from build123d import *

# Parameters (mm, degrees)
BOSS_EXTRU_1_DEPTH      = 5
ESQUISSE2_W             = 5
ESQUISSE2_H             = 28
ESQUISSE2_W_2           = 47.6
ESQUISSE2_H_2           = 5
ESQUISSE2_H_3           = 33
ENL_V_MAT_EXTRU_1_DEPTH = 5


with BuildPart() as part:
    # Esquisse1 → Boss.-Extru.1 (new body)
    with BuildSketch(Plane.XY):
        Polygon((0, 0), (0, 145), (238, 170), (238, 5), (238, 0), align=None)
    extrude(amount=BOSS_EXTRU_1_DEPTH)

    # Esquisse2 → Enlèv. mat.-Extru.1 (cut)
    with BuildSketch(Plane.XY.offset(5)):
        with Locations((2.5, 42)):
            Rectangle(ESQUISSE2_W, ESQUISSE2_H)
        with Locations((2.5, 98)):
            Rectangle(ESQUISSE2_W, ESQUISSE2_H)
        with Locations((71.4, 2.5)):
            Rectangle(ESQUISSE2_W_2, ESQUISSE2_H_2)
        with Locations((166.6, 2.5)):
            Rectangle(ESQUISSE2_W_2, ESQUISSE2_H_2)
        with Locations((235.5, 115.5)):
            Rectangle(ESQUISSE2_W, ESQUISSE2_H_3)
        with Locations((235.5, 49.5)):
            Rectangle(ESQUISSE2_W, ESQUISSE2_H_3)
    extrude(amount=-ENL_V_MAT_EXTRU_1_DEPTH, mode=Mode.SUBTRACT)


solid = part.part
Part model, mm, in its own coordinate system. A direction names the side the tool comes from. Round coordinates to 2 decimals unless told otherwise and drop trailing zeros. Write each loop counter-clockwise with the first axis right and the second up, starting at its lowest first coordinate (ties: lowest second). Pieces come first, ordered by that corner, then holes. Notation, with made-up numbers: M 55,-22 L 108,-22 A24 ccw 108,2 Z; hole C -25.75,51.25 d11. An arc over 180 degrees is marked long. Return JSON: item names as keys, results as strings. Group by question number.
(1) Pin check, flat tips, straight feed: pin 1 Ø1.5 at (x, z) = (235, 2) entering from +Y; pin 2 Ø1.5 at (x, z) = (2.5, 1.5) entering from +Y; pin 3 Ø1 at (x, z) = (57.5, 3) entering from +Y. Stop position of each tip, or through.
(2) Two-plate mould, pull along Y, no slides. Class faces 4 (the face through (238, 151, 2)), 5 (the face through (215, 0, 2)), 6 (the face through (233, 49, 3)), 7 (the face through (235, 33, 3)): +Y half, -Y half, draft (parallel to the pull), parting line (faces both ways), or undercut.
(3) Saw through at B-B on y = 39.5. Write the cut outline in (x, z).
(4) Drill centre lines: probe 1 along X at (y, z) = (91.5, 0.8); probe 2 along X at (y, z) = (119.5, 1.95); probe 3 along Y at (x, z) = (97, 3.05). Where is each one in solid material? Low to high.
(5) Saw through at A-A on z = 4.1. Write the cut outline in (x, y).
(6) Which spindle directions (+Z, -Z, +X, -X, +Y, -Y) get a long thin tool onto all of the face, cutting with end or side? Do faces 1 (the face through (47.6, 2, 3)), 2 (the face through (5, 42, 3)), 3 (the face through (235, 66, 3)). Say none if no direction does.
(7) Saw through at C-C on x = 196.5. Write the cut outline in (y, z), then the cut area to 3 significant figures.
Returned:
{
 "1": {"pin 1": "y = 169.76", "pin 2": "y = 145.34", "pin 3": "y = 151.09"},
 "2": {"face 4": "draft", "face 5": "-Y half", "face 6": "undercut", "face 7": "undercut"},
 "3": {"outline": "M 5,0 L 233,0 L 233,5 L 5,5 Z"},
 "4": {"probe 1": "5 to 238", "probe 2": "0 to 233", "probe 3": "0 to 155.19"},
 "5": {"outline": "M 0,0 L 47.6,0 L 47.6,5 L 95.2,5 L 95.2,0 L 142.8,0 L 142.8,5 L 190.4,5 L 190.4,0 L 238,0 L 238,33 L 233,33 L 233,66 L 238,66 L 238,99 L 233,99 L 233,132 L 238,132 L 238,170 L 0,145 L 0,112 L 5,112 L 5,84 L 0,84 L 0,56 L 5,56 L 5,28 L 0,28 Z"},
 "6": {"face 1": "+Z, -Z, -Y", "face 2": "+Z, -Z, -X", "face 3": "+Z, -Z, +X"},
 "7": {"outline": "M 0,0 L 165.64,0 L 165.64,5 L 0,5 Z", "area": "828 mm²"}
}
